For this review, use the dimensioned drawing (mm, ordinates from the lowest corner) and the shaded views. A direction names the side the tool comes from. Round coordinates to 2 decimals unless told otherwise and drop trailing zeros. Order: outer loops, then holes, each group sorted by start corner. A loop starts at its lowest first (then second) coordinate and runs counter-clockwise, first axis right, second up. Notation, with made-up numbers: (-14.75, 33) - (3.25, 33) arc R21 cw to (3.25, 71) - close; hole circle Ø1 at (-25.75, -27). An arc over 180 degrees is marked (long way). Write item = value, one per line.
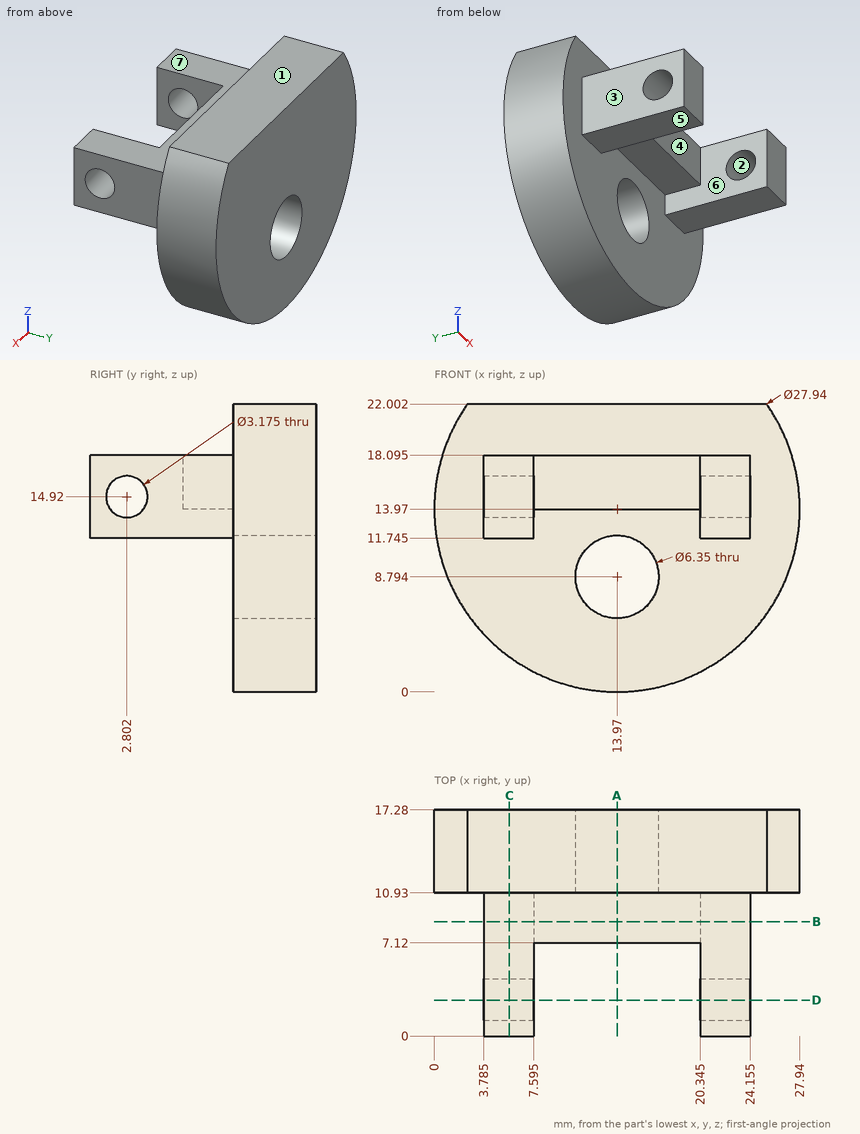
1) For the marked faces 4, 5, 6 and 7, list the 3-axis set-ups (+Z, -Z, +X, -X, +Y, -Y) from which the entire face can be reached by the end or side of a thin tool; tool diameter is ignored.
Findings:
face_4 = +Z, -Z, -Y
face_5 = -Z, +X, -X, -Y
face_6 = -Z, -Y
face_7 = +Z, +X, -X, -Y
2) We need section A-A on x = 13.97. Write out the cut boundary in (y, z) (1 decimal).
Findings:
outline = (7.1, 14) - (10.9, 14) - (10.9, 12) - (17.3, 12) - (17.3, 22) - (10.9, 22) - (10.9, 18.1) - (7.1, 18.1) - close; (10.9, 0) - (17.3, 0) - (17.3, 5.6) - (10.9, 5.6) - close
3) We need section D-D on y = 2.75. Write out the cut boundary in (x, z) (1 decimal).
Findings:
outline = (3.8, 11.7) - (7.6, 11.7) - (7.6, 13.3) - (3.8, 13.3) - close; (3.8, 16.5) - (7.6, 16.5) - (7.6, 18.1) - (3.8, 18.1) - close; (20.3, 11.7) - (24.2, 11.7) - (24.2, 13.3) - (20.3, 13.3) - close; (20.3, 16.5) - (24.2, 16.5) - (24.2, 18.1) - (20.3, 18.1) - close
4) We need section B-B on y = 8.75. Write out the cut boundary in (x, z) (3 decimals).
Findings:
outline = (3.785, 11.745) - (7.595, 11.745) - (7.595, 13.97) - (20.345, 13.97) - (20.345, 11.745) - (24.155, 11.745) - (24.155, 18.095) - (3.785, 18.095) - close
5) We need section C-C on x = 5.75. Write out the cut boundary in (y, z) (1 decimal), and give its area (3 significant figures).
Findings:
outline = (0, 11.7) - (10.9, 11.7) - (10.9, 2.7) - (17.3, 2.7) - (17.3, 22) - (10.9, 22) - (10.9, 18.1) - (0, 18.1) - close; hole circle Ø3.2 at (2.8, 14.9)
area = 184 mm^2
6) To check wall thickness, follow L1, parallel to Z at x = 13.97, y = 15.25; L2, parallel to Y at x = 14.25, z = 14.75; L3, parallel to Y at x = 9.5, z = 18.5. State the ranges of each line that lie inside material, in increasing order. Write a range as from..to.
Findings:
L1 = 0..5.62, 11.97..22
L2 = 7.12..17.28
L3 = 10.93..17.28
7) Clearance check with flat-ended pins moving along their axes: pin 1 Ø4 at (y, z) = (2.8, 14.92) entering from +X (3 decimals); pin 2 Ø4 at (x, y) = (6.5, 5.5) entering from -Z (3 decimals); pin 3 Ø1.5 at (y, z) = (15.5, 4.5) entering from +X; pin 4 Ø4 at (x, z) = (13.97, 8.79) entering from +Y. State where each tip first meets the part, or that it passes through.
Findings:
pin_1 = 24.155
pin_2 = 11.745
pin_3 = 24.88
pin_4 = through
8) The part is to be moulded in two halves that separate along Z. For the marked faces 1, 2 and 3, say which applies: released by +Z, released by -Z, zero draft, split by the parting line, or undercut.
Findings:
face_1 = released by +Z
face_2 = undercut
face_3 = zero draft
